Job drawing, mm, ordinate dimensions from the low corner. One solid piece. A direction names the side the tool comes from. Give positions to 0.01 mm unless a question says otherwise; leave off trailing zeros. Order: outer loops, then holes, each group sorted by start corner. A loop starts at its lowest first (then second) coordinate and runs counter-clockwise, first axis right, second up. Notation, with made-up numbers: (50.5, -39.5) - (73.5, -39.5) arc R27 cw to (73.5, -5.5) - close; hole circle Ø3 at (38, 45). An arc over 180 degrees is marked (long way). Write each question's results on one line, items separated by ' | '. Start each with the question number.
1) Cut at C-C on y = 28.5. List the corners of the cut face in (x, z), plus the area to 3 significant figures.
2) Cut at B-B on x = 6. List the corners of the cut face in (y, z).
3) Cut at A-A on z = 5. List the corners of the cut face in (x, y).
4) Drill centre lines: line 1 along Z through (x, y) = (3, 15); line 2 along Y through (x, z) = (7.75, 12.25); line 3 along Y through (x, z) = (2.75, 3). Where is each one in solid material? Low to high. Write a range as from..to.
5) Tool access for the marked faces 1, 2 and 3: list every direction of +Z, -Z, +X, -X, +Y, -Y with a clear straight run to the whole face (end or side of a thin tool).
6) Cut at D-D on x = 2. List the corners of the cut face in (y, z), plus the area to 3 significant figures.
7) Drop a flat-ended pin along its axis: pin 1 Ø2.5 at (x, z) = (3.5, 13.5) entering from +Y. Give the stop position or say it passes through.
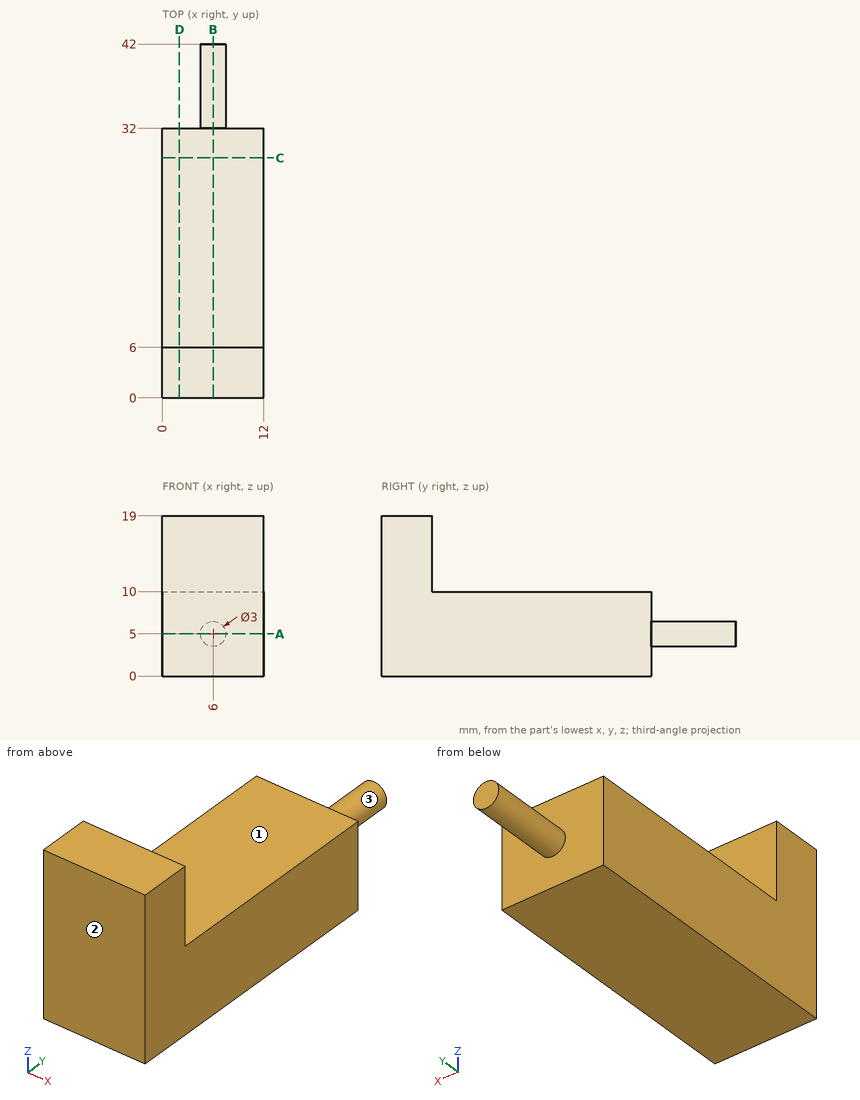
Results:
1) outline: (0, 0) - (12, 0) - (12, 10) - (0, 10) - close | area: 120 mm^2
2) outline: (0, 0) - (32, 0) - (32, 3.5) - (42, 3.5) - (42, 6.5) - (32, 6.5) - (32, 10) - (6, 10) - (6, 19) - (0, 19) - close
3) outline: (0, 0) - (12, 0) - (12, 32) - (7.5, 32) - (7.5, 42) - (4.5, 42) - (4.5, 32) - (0, 32) - close
4) line 1: 0..10 | line 2: 0..6 | line 3: 0..32
5) face 1: +Z, +X, -X, +Y | face 2: +Z, -Z, +X, -X, -Y | face 3: +Y
6) outline: (0, 0) - (32, 0) - (32, 10) - (6, 10) - (6, 19) - (0, 19) - close | area: 374 mm^2
7) pin 1: y = 6
